Verification items for the finished model (mm, model axes). A direction names the side the tool comes from. Give positions to 0.01 mm unless a question says otherwise; leave off trailing zeros. Write each loop counter-clockwise with the first axis right and the second up, starting at its lowest first coordinate (ties: lowest second). Pieces come first, ordered by that corner, then holes. Notation, with made-up numbers: (-6.75, -3.75) - (47.25, -3.75) arc R26 ccw to (47.25, 19.25) - close; hole circle Ø9 at (-38.5, -25). An arc over 180 degrees is marked (long way). Answer as a JSON object with one key per item and string values. Group by question number.
Item 1: Go/stop test with flat-tipped pins: pin 1 (3 mm diameter, centred on y = 7, z = -11, fed in from +X); pin 2 (10 mm diameter, centred on x = -5.5, z = 6, fed in from -Y). Record where each tip stops, or that it passes through.
Item 2: Sectioned sample at B-B, the plane z = 0. Record the boundary of the cut face in (x, y) (3 decimals).
Item 3: Tool access check on faces 5 (the face through (-7.638, 1.726, -5.857)), 6 (the face through (-11.587, 4.056, -0.023)). Record the directions out of +Z, -Z, +X, -X, +Y, -Y that give a thin tool (end or side, any length) a straight path to the whole face; none if there is none.
Item 4: Sectioned sample at C-C, the plane x = 0. Record the boundary of the cut face in (y, z) (3 decimals).
Item 5: Sectioned sample at A-A, the plane y = 1.5. Count the separate pieces of the cut face and the enclosed holes in it, and give its area (3 significant figures).
Item 6: Scan lines: line 1 along X through (y, z) = (5.95, 0); line 2 along X through (y, z) = (7.25, 10.5); line 3 along Y through (x, z) = (-7.25, 1.5). Record each from-to range of solid material in increasing order. Write a range as [from, to].
Item 7: Draft check along Z on faces 1 (the face through (9, 0, 4)), 2 (the face through (-5.96, 5.47, -1.88)), 3 (the face through (-7, 4, 10)), 4 (the face through (0.5, 3.9, -13.3)). Enter one of: +Z half, -Z half, draft (parallel to the pull), parting line (faces both ways), or undercut.
Item 8: Sectioned sample at D-D, the plane y = 6.5. Record the boundary of the cut face in (x, z).
Autodesk Inventor part; units mm, degrees
ref_plane "YZ Plane" through (0, 0, 0) normal (1, 0, 0) x (0, 1, 0)
ref_plane "XZ Plane" through (0, 0, 0) normal (0, 1, 0) x (-1, 0, 0)
ref_plane "XY Plane" through (0, 0, 0) normal (0, 0, 1) x (1, 0, 0)
sketch "Sketch1" plane through (0, 0, 0) normal (0, 1, 0) x (-1, 0, 0)
  circle A0 centre (0, 0) radius 6.25
  circle A1 centre (0, -15.75) radius 2.5
  circle A2 centre (0, 15.75) radius 2.5
  line L0 (0, 0) -> (0, -24)
  line L1 (0, 0) -> (0, 24)
  line L2 (0, 0) -> (12, 0)
  line L3 (0, 0) -> (-12, 0)
  line L4 (0, 24) -> (12, 0)
  line L5 (12, 0) -> (0, -24)
  line L6 (0, -24) -> (-12, 0)
  line L7 (-12, 0) -> (0, 24)
  dimension "d0" = 12.5
  dimension "d1" = 5
  dimension "d2" = 5
  dimension "d3" = 15.75
  dimension "d4" = 15.75
  dimension "d5" = 24
  dimension "d6" = 24
  dimension "d7" = 12
  dimension "d8" = 12
extrude "Extrusion1" add sketch "Sketch1" along normal blind 8 contours L2 L5 L0 A1 A0 | A0 L1 A2 L4 L2 | A0 L3 L7 L1 A2 | L0 A1 L6 L3 A0
fillet "Fillet1" radius 3.5 4 edges at (0, 4, 24) (0, 4, -24) (12, 4, 0) (-12, 4, 0)
sketch "Sketch2" plane through (0, 0, 0) normal (0, -1, 0) x (1, 0, 0)
  circle A0 centre (0, 0) radius 6.25
  circle A1 centre (0, 0) radius 9.625
  dimension "d12" = 19.25
extrude "Extrusion2" cut sketch "Sketch2" against normal blind 3.5
fillet "Fillet2" radius 0.5 1 edges at (6.25, 8, 0)
properties part number "no-filter-inlet"
Geometry check:
{
 "1": {"pin 1": "x = 7.25", "pin 2": "y = 0"},
 "2": {"outline": "(-11.587, 0) - (-9.625, 0) - (-9.625, 3.5) - (-6.25, 3.5) - (-6.25, 7.5) arc R0.5 ccw to (-6.75, 8) - (-11.587, 8) - close; (6.25, 3.5) - (9.625, 3.5) - (9.625, 0) - (11.587, 0) - (11.587, 8) - (6.75, 8) arc R0.5 ccw to (6.25, 7.5) - close"},
 "3": {"face 5": "-Y", "face 6": "-X, +Y, -Y"},
 "4": {"outline": "(0, -19.674) - (8, -19.674) - (8, -18.25) - (0, -18.25) - close; (0, -13.25) - (8, -13.25) - (8, -6.75) arc R0.5 ccw to (7.5, -6.25) - (3.5, -6.25) - (3.5, -9.625) - (0, -9.625) - close; (0, 9.625) - (3.5, 9.625) - (3.5, 6.25) - (7.5, 6.25) arc R0.5 ccw to (8, 6.75) - (8, 13.25) - (0, 13.25) - close; (0, 18.25) - (8, 18.25) - (8, 19.674) - (0, 19.674) - close"},
 "5": {"separate pieces": "1", "enclosed holes": "3", "area": "223 mm^2"},
 "6": {"line 1": "[-11.59, -6.25], [6.25, 11.59]", "line 2": "[-6.75, 6.75]", "line 3": "[3.5, 8]"},
 "7": {"face 1": "draft", "face 2": "undercut", "face 3": "+Z half", "face 4": "undercut"},
 "8": {"outline": "(-11.22, -1.57) - (-3.13, -17.74) arc R3.5 ccw to (3.13, -17.74) - (11.22, -1.57) arc R3.5 ccw to (11.22, 1.57) - (3.13, 17.74) arc R3.5 ccw to (-3.13, 17.74) - (-11.22, 1.57) arc R3.5 ccw to start; hole circle Ø12.5 at (0, 0); hole circle Ø5 at (0, -15.75); hole circle Ø5 at (0, 15.75)"}
}
